Print and shaded views of the part. All mm, measured from the part's lowest x, y and z. A direction names the side the tool comes from. Give positions to 0.01 mm unless a question says otherwise; leave off trailing zeros. Loops run counter-clockwise (first coordinate to the right, second up) from the corner with the lowest first, then second, coordinate; pieces in that order, holes last. Notation, with made-up numbers: (0, 2) -> (29, 2) arc R16 ccw to (29, 27) -> close; hole circle Ø2 at (-0.5, 40). An arc over 180 degrees is marked (long way). Answer as a JSON object with one key per item and string values. Group by question number.
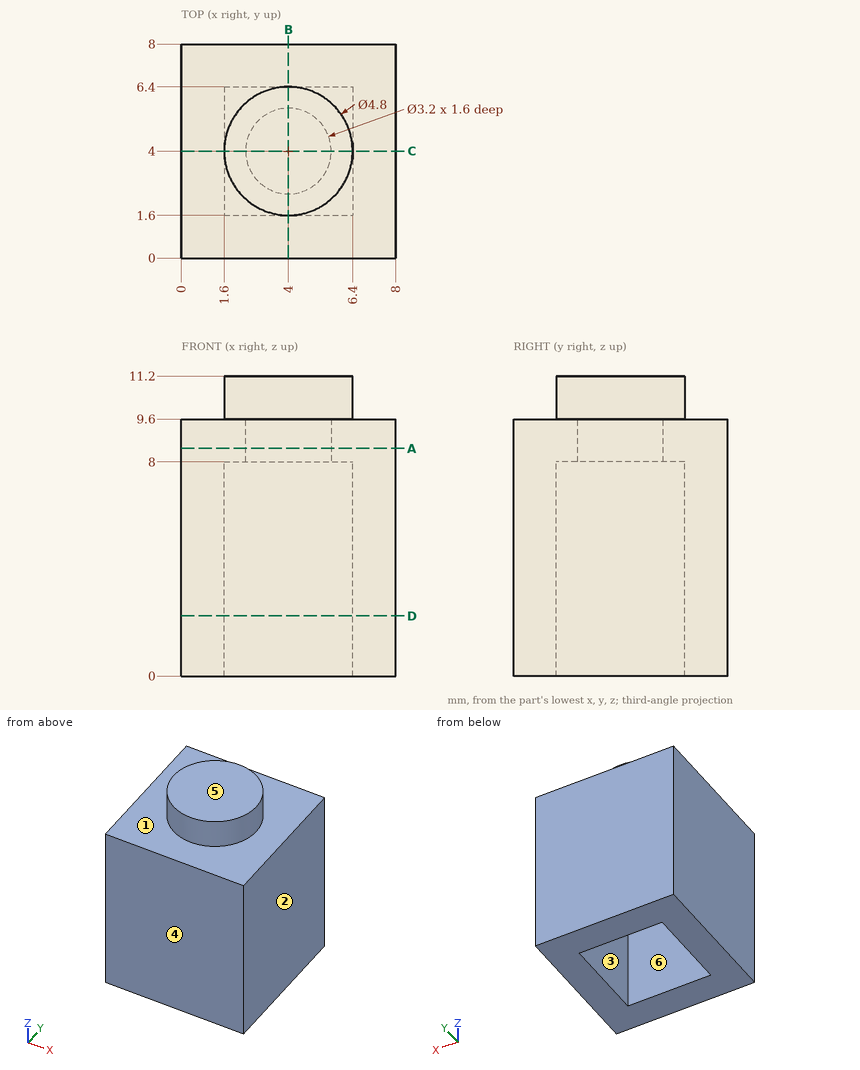
(1) Saw through at A-A on z = 8.5. List the corners of the cut face in (x, y).
(2) Probe line 1 along Y through (x, z) = (4, 9.15); line 2 along X through (y, z) = (2, 3). List the from-to ranges inside material, lowest first. Write a range as [from, to].
(3) Saw through at B-B on x = 4. List the corners of the cut face in (y, z), plus the area to 3 significant figures.
(4) Pin check, flat tips, straight feed: pin 1 (3 mm diameter, centred on x = 4, y = 4, fed in from -Z); pin 2 (1 mm diameter, centred on x = 7, y = 1.5, fed in from +Z); pin 3 (2.5 mm diameter, centred on x = 3, y = 3.5, fed in from -Z). Stop position of each tip, or through.
(5) 3-axis set-ups, long thin cutter, end or side, ignore diameter. For the marked faces 1, 2 and 3: which of +Z, -Z, +X, -X, +Y, -Y reach the whole face in a straight line?
(6) Pull direction Y, two halves, no side cores. Call the marked faces 4, 5 and 6: pulls with the +Y half, pulls with the -Y half, needs draft (parallel to the pull), parting line crosses it, or undercut.
(7) Saw through at D-D on z = 2.25. List the corners of the cut face in (x, y), plus the area to 3 significant figures.
Calculated:
{
 "1": {"outline": "(0, 0) -> (8, 0) -> (8, 8) -> (0, 8) -> close; hole circle Ø3.2 at (4, 4)"},
 "2": {"line 1": "y = [0, 2.4], [5.6, 8]", "line 2": "x = [0, 1.6], [6.4, 8]"},
 "3": {"outline": "(0, 0) -> (1.6, 0) -> (1.6, 8) -> (2.4, 8) -> (2.4, 9.6) -> (5.6, 9.6) -> (5.6, 8) -> (6.4, 8) -> (6.4, 0) -> (8, 0) -> (8, 9.6) -> (6.4, 9.6) -> (6.4, 11.2) -> (1.6, 11.2) -> (1.6, 9.6) -> (0, 9.6) -> close", "area": "41.0 mm^2"},
 "4": {"pin 1": "stops at z = 9.6", "pin 2": "stops at z = 9.6", "pin 3": "stops at z = 8"},
 "5": {"face 1": "+Z", "face 2": "+Z, -Z, +X, +Y, -Y", "face 3": "-Z"},
 "6": {"face 4": "pulls with the -Y half", "face 5": "needs draft", "face 6": "undercut"},
 "7": {"outline": "(0, 0) -> (8, 0) -> (8, 8) -> (0, 8) -> close; hole (1.6, 1.6) -> (6.4, 1.6) -> (6.4, 6.4) -> (1.6, 6.4) -> close", "area": "41.0 mm^2"}
}
